```python
from build123d import *

# Parameters (mm, degrees)
BOSS_EXTRUDE2_DEPTH = 25.4
SKETCH3_W           = 61.065778348
SKETCH3_H           = 22.225
CUT_EXTRUDE2_DEPTH  = 69.777192209
SKETCH4_R           = 3.302
CUT_EXTRUDE3_DEPTH  = 49.382028551


with BuildPart() as part:
    # Sketch1 → Boss-Extrude2 (new body)
    with BuildSketch(Plane(origin=(0, 0, 0), x_dir=(1, 0, 0), z_dir=(0, 1, 0))):
        with BuildLine():
            Line((0, 0), (28.222222222, 0))
            Line((28.222222222, 0), (28.222222222, 14.111111111))
            Line((28.222222222, 14.111111111), (15.875, 14.111111111))
            ThreePointArc((15.875, 14.111111111), (0, 29.986111111), (-15.875, 14.111111111))
            Line((-15.875, 14.111111111), (-28.222222222, 14.111111111))
            Line((-28.222222222, 14.111111111), (-28.222222222, 0))
            Line((-28.222222222, 0), (0, 0))
        make_face()
    extrude(amount=BOSS_EXTRUDE2_DEPTH)

    # Sketch3 → Cut-Extrude2 (cut, through all)
    with BuildSketch(Plane(origin=(28.222222222, 0, 0), x_dir=(0, 0, -1), z_dir=(1, 0, 0))):
        with Locations((32.120389174, 12.7)):
            Rectangle(SKETCH3_W, SKETCH3_H)
    extrude(amount=-CUT_EXTRUDE2_DEPTH, mode=Mode.SUBTRACT)

    # Sketch4 → Cut-Extrude3 (cut, through all)
    with BuildSketch(Plane(origin=(0, 25.4, 0), x_dir=(1, 0, 0), z_dir=(0, 1, 0))):
        with Locations(Location((0, 17.78, 0), (0, 0, 270))):
            Circle(SKETCH4_R)
    extrude(amount=-CUT_EXTRUDE3_DEPTH, mode=Mode.SUBTRACT)


solid = part.part
```
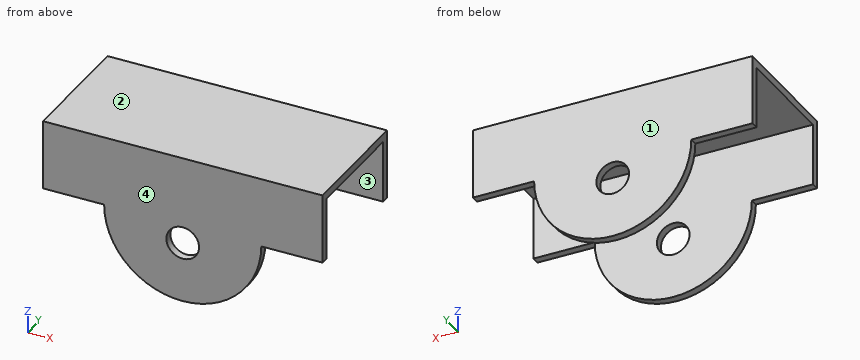
Design review of the part built by this model. Coordinates are the model's own, in mm. Face numbers are marked on the shaded views. Give positions to 0.01 mm unless a question says otherwise; leave off trailing zeros. Write each loop counter-clockwise with the first axis right and the second up, starting at its lowest first coordinate (ties: lowest second). Pieces come first, ordered by that corner, then holes.
(1) Clearance check with flat-ended pins moving along their axes: pin 1 Ø0.5 at (x, y) = (-22, 24.5) entering from -Z; pin 2 Ø1 at (x, y) = (15, 13) entering from +Z; pin 3 Ø6.5 at (x, y) = (-10.5, 9.5) entering from -Z. State where each tip first meets the part, or that it passes through.
Checked values:
pin 1: stops at z = -14.11
pin 2: stops at z = 0
pin 3: stops at z = -1.59
(2) Wall thickness on line 1 along Y through (x, z) = (19, -5.5); line 2 along Z through (x, y) = (5, 13.5); line 3 along X through (y, z) = (1.1, -17.78): over which ranges is each line inside the solid? List them lowest first.
Checked values:
line 1: y = 0 to 1.59, 23.81 to 25.4
line 2: z = -1.59 to 0
line 3: x = -15.45 to -3.3, 3.3 to 15.45
(3) Mouldability with a two-part tool opening along Y and no side actions: class the marked faces 1, 2, 3 and 4 as +Y half, -Y half, draft (parallel to the pull), parting line (faces both ways), or undercut.
Checked values:
face 1: +Y half
face 2: draft
face 3: undercut
face 4: -Y half
(4) Add section A-A (x = 0). Give the boundary of the cut face in (y, z).
Checked values:
outline: (0, -29.99) - (1.59, -29.99) - (1.59, -21.08) - (0, -21.08) - close; (0, -14.48) - (1.59, -14.48) - (1.59, -1.59) - (23.81, -1.59) - (23.81, -14.48) - (25.4, -14.48) - (25.4, 0) - (0, 0) - close; (23.81, -29.99) - (25.4, -29.99) - (25.4, -21.08) - (23.81, -21.08) - close
(5) Add section B-B (z = -12.25). Give the boundary of the cut face in (x, y), and give its area (3 significant figures).
Checked values:
outline: (-28.22, 0) - (28.22, 0) - (28.22, 1.59) - (-28.22, 1.59) - close; (-28.22, 23.81) - (28.22, 23.81) - (28.22, 25.4) - (-28.22, 25.4) - close
area: 179 mm2
(6) Add section D-D (x = -23.5). Give the boundary of the cut face in (y, z), and give its area (3 significant figures).
Checked values:
outline: (0, -14.11) - (1.59, -14.11) - (1.59, -1.59) - (23.81, -1.59) - (23.81, -14.11) - (25.4, -14.11) - (25.4, 0) - (0, 0) - close
area: 80.1 mm2
(7) Add section C-C (z = -17.78). Give the boundary of the cut face in (x, y).
Checked values:
outline: (-15.45, 0) - (-3.3, 0) - (-3.3, 1.59) - (-15.45, 1.59) - close; (-15.45, 23.81) - (-3.3, 23.81) - (-3.3, 25.4) - (-15.45, 25.4) - close; (3.3, 0) - (15.45, 0) - (15.45, 1.59) - (3.3, 1.59) - close; (3.3, 23.81) - (15.45, 23.81) - (15.45, 25.4) - (3.3, 25.4) - close
